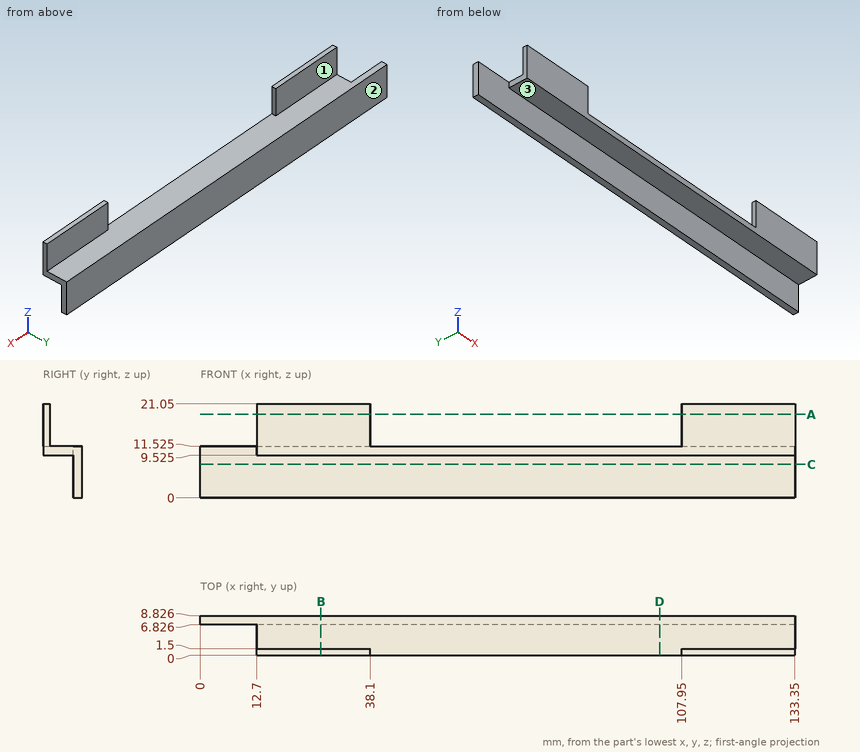
Part print with two shaded views. Sizes in mm from the minimum x, y, z corner. A direction names the side the tool comes from. Round coordinates to 2 decimals unless told otherwise and drop trailing zeros. Loops run counter-clockwise (first coordinate to the right, second up) from the corner with the lowest first, then second, coordinate; pieces in that order, holes last. Notation, with made-up numbers: M 71.5,60.5 L 119.5,60.5 A29 cw 119.5,87.5 Z; hole C 72,88 d1. An arc over 180 degrees is marked long. Put each result on its own line as item: value. Start each with the question number.
Item 1: Cut at A-A (z = 18.75). List the corners of the cut face in (x, y).
Item 2: Drop flat-ended pins along their axis: P1, Ø2, axis at x = 66.5, z = 3.5, coming from the -Y side; P2, Ø3, axis at x = 26.5, z = 15.5, coming from the +Y side; P3, Ø2, axis at y = 2, z = 12.5, coming from the -X side. Give the stop position or say it passes through.
Item 3: Cut at D-D (x = 103). List the corners of the cut face in (y, z) (3 decimals), then the cut area to 3 significant figures.
Item 4: Cut at B-B (x = 27). List the corners of the cut face in (y, z) (3 decimals), then the cut area to 3 significant figures.
Item 5: Cut at C-C (z = 7.5). List the corners of the cut face in (x, y), then the cut area to 3 significant figures.
Item 6: Drill centre lines: line 1 along Y through (x, z) = (112, 6.25); line 2 along Z through (x, y) = (126.5, 7.25) (3 decimals); line 3 along Z through (x, y) = (18, 3.5) (3 decimals). Where is each one in solid material? Low to high.
Item 7: 3-axis set-ups, long thin cutter, end or side, ignore diameter. For the marked faces 1, 2 and 3: which of +Z, -Z, +X, -X, +Y, -Y reach the whole face in a straight line?
Answer block:
1. outline: M 12.7,0 L 38.1,0 L 38.1,1.5 L 12.7,1.5 Z; M 107.95,0 L 133.35,0 L 133.35,1.5 L 107.95,1.5 Z
2. P1: y = 6.83
2. P2: y = 1.5
2. P3: x = 12.7
3. outline: M 0,9.525 L 6.826,9.525 L 6.826,0 L 8.826,0 L 8.826,11.525 L 0,11.525 Z
3. area: 36.7 mm2
4. outline: M 0,9.525 L 6.826,9.525 L 6.826,0 L 8.826,0 L 8.826,11.525 L 1.5,11.525 L 1.5,21.05 L 0,21.05 Z
4. area: 51.0 mm2
5. outline: M 0,6.83 L 133.35,6.83 L 133.35,8.83 L 0,8.83 Z
5. area: 267 mm2
6. line 1: 6.83 to 8.83
6. line 2: 0 to 11.525
6. line 3: 9.525 to 11.525
7. face 1: +Z, +X, -X, +Y
7. face 2: +Z, -Z, +X, -X, +Y
7. face 3: -Z, +X, -X, -Y
